Part model, mm, in its own coordinate system. A direction names the side the tool comes from. Coordinates: 2 decimals unless noted, no trailing zeros. Loops run counter-clockwise (first coordinate to the right, second up) from the corner with the lowest first, then second, coordinate; pieces in that order, holes last. Notation, with made-up numbers: M 28.5,-0.5 L 51.5,-0.5 A23 cw 51.5,30.5 Z; hole C 54,19.25 d7. An arc over 180 degrees is marked long. Use a Markdown table: item, result. Add a question column.
1) Tool access for faces 5 (the flat face through (1.22, -0.5, 0)), 6 (the flat face through (-2, 1.6, 1)), 7 (the flat face through (-1.22, -0.5, 0)), 8 (the flat face through (0, -1, 0)), 9 (the flat face through (0, -0.5, 2.22)): list every direction of +Z, -Z, +X, -X, +Y, -Y with a clear straight run to the whole face (end or side of a thin tool).
2) Band-saw the part on B-B (x = 1.5). List the corners of the cut face in (y, z).
3) Band-saw the part on A-A (z = 0). List the corners of the cut face in (x, y).
4) Pin check, flat tips, straight feed: pin 1 Ø1.5 at (x, y) = (-1, 0) entering from -Z; pin 2 Ø0.8 at (x, y) = (-0.5, -0.5) entering from +Z; pin 3 Ø1.5 at (y, z) = (0.5, 2) entering from -X. Stop position of each tip, or through.
5) Pull direction Z, two halves, no side cores. Call faces 1 (the cylindrical face through (-3.417, 0.74, -0.759)), 2 (the flat face through (0, -0.5, -2.22)), 3 (the flat face through (0, 1.5, 0)), 4 (the flat face through (0, 1.6, -2)): released by +Z, released by -Z, zero draft, split by the parting line, or undercut.
6) Band-saw the part on C-C (y = 0.8). List the corners of the cut face in (x, z).
7) Wall check: probe 1 along Y at (x, z) = (1.25, -1.25); probe 2 along X at (y, z) = (-0.2, 1.75); probe 3 along Y at (x, z) = (-0.25, 1.5). Give the ranges that are in metal, low to high. Write a range as from..to.
8) Band-saw the part on D-D (z = 2.5). List the corners of the cut face in (x, y) (3 decimals).
from build123d import *

# Parameters (mm, degrees)
SKETCH1_R           = 3.5
SKETCH1_W           = 2.44
SKETCH1_H           = 4.44
BOSS_EXTRUDE1_DEPTH = 1.5
SKETCH1_3_W         = 2.44
SKETCH1_3_H         = 4.44
BOSS_EXTRUDE2_DEPTH = 1
SKETCH2_W           = 1.27
SKETCH2_H           = 1.27
BOSS_EXTRUDE3_DEPTH = 0.1


with BuildPart() as part:
    # Sketch1 → Boss-Extrude1 (new body)
    # profile 1 of 2: a face of its own
    with BuildSketch(Plane(origin=(0, 0, 0), x_dir=(1, 0, 0), z_dir=(0, 1, 0))):
        with Locations(Location((0, 0, 0), (0, 0, 270))):
            Circle(SKETCH1_R)
        Rectangle(SKETCH1_W, SKETCH1_H, mode=Mode.SUBTRACT)
    # profile 2 of 2: a face of its own
    with BuildSketch(Plane(origin=(0, 0, 0), x_dir=(1, 0, 0), z_dir=(0, 1, 0))):
        Rectangle(SKETCH1_W, SKETCH1_H)
    extrude(amount=BOSS_EXTRUDE1_DEPTH)

    # Sketch1_3 → Boss-Extrude2 (add)
    with BuildSketch(Plane(origin=(0, 0, 0), x_dir=(1, 0, 0), z_dir=(0, 1, 0))):
        Rectangle(SKETCH1_3_W, SKETCH1_3_H)
    extrude(amount=-BOSS_EXTRUDE2_DEPTH)

    # Sketch2 → Boss-Extrude3 (add)
    with BuildSketch(Plane(origin=(0, 1.5, 0), x_dir=(1, 0, 0), z_dir=(0, 1, 0))):
        with Locations((0, 2.3)):
            Rectangle(SKETCH2_W, SKETCH2_H)
        Polygon((2.22428456, 2.017426131), (1.124432297, 1.382426131), (1.759432297, 0.282573869), (2.85928456, 0.917573869), align=None)
        Polygon((2.85928456, -0.917573869), (1.759432297, -0.282573869), (1.124432297, -1.382426131), (2.22428456, -2.017426131), align=None)
        with Locations((0, -2.3)):
            Rectangle(SKETCH2_W, SKETCH2_H)
        Polygon((-2.22428456, -2.017426131), (-1.124432297, -1.382426131), (-1.759432297, -0.282573869), (-2.85928456, -0.917573869), align=None)
        Polygon((-2.85928456, 0.917573869), (-1.759432297, 0.282573869), (-1.124432297, 1.382426131), (-2.22428456, 2.017426131), align=None)
    extrude(amount=BOSS_EXTRUDE3_DEPTH)


solid = part.part
Entries:
| question | item | result |
|---|---|---|
| 1 | face 5 | +Z, -Z, +X, -Y |
| 1 | face 6 | +Z, -Z, +X, -X, +Y |
| 1 | face 7 | +Z, -Z, -X, -Y |
| 1 | face 8 | +Z, -Z, +X, -X, -Y |
| 1 | face 9 | +Z, +X, -X, -Y |
| 2 | outline | M 0,-3.16 L 1.5,-3.16 L 1.5,-1.6 L 1.6,-1.6 L 1.6,-0.73 L 1.5,-0.73 L 1.5,0.73 L 1.6,0.73 L 1.6,1.6 L 1.5,1.6 L 1.5,3.16 L 0,3.16 Z |
| 3 | outline | M -3.5,0 L -1.22,0 L -1.22,-1 L 1.22,-1 L 1.22,0 L 3.5,0 L 3.5,1.5 L -3.5,1.5 Z |
| 4 | pin 1 | z = -3.49 |
| 4 | pin 2 | z = 2.22 |
| 4 | pin 3 | x = -3.27 |
| 5 | face 1 | split by the parting line |
| 5 | face 2 | released by -Z |
| 5 | face 3 | undercut |
| 5 | face 4 | zero draft |
| 6 | outline | C 0,0 d7 |
| 7 | probe 1 | 0..1.6 |
| 7 | probe 2 | -1.22..1.22 |
| 7 | probe 3 | -1..1.5 |
| 8 | outline | M -2.449,0 L 2.449,0 L 2.449,1.5 L 0.635,1.5 L 0.635,1.6 L -0.635,1.6 L -0.635,1.5 L -2.449,1.5 Z |
